For this review, take the finished solid that the model builds, in its own axes (mm). A direction names the side the tool comes from. Round coordinates to 2 decimals unless told otherwise and drop trailing zeros. Order: outer loops, then holes, each group sorted by start corner. A loop starts at its lowest first (then second) coordinate and runs counter-clockwise, first axis right, second up.
Autodesk Inventor part; units mm, degrees
ref_plane "YZ Plane" through (0, 0, 0) normal (1, 0, 0) x (0, 1, 0)
ref_plane "XZ Plane" through (0, 0, 0) normal (0, 1, 0) x (-1, 0, 0)
ref_plane "XY Plane" through (0, 0, 0) normal (0, 0, 1) x (1, 0, 0)
sketch "Sketch1" plane through (0, 0, 0) normal (0, 0, 1) x (1, 0, 0)
  line L0 (0, 0) -> (-34.798, 0)
  line L1 (-34.798, 0) -> (-34.798, -56.642)
  line L2 (0, -12.7) -> (-28.448, -12.7)
  line L3 (-28.448, -12.7) -> (-28.448, -25.654)
  line L4 (-28.448, -25.654) -> (0, -25.654)
  line L5 (0, -56.642) -> (0, -25.654)
  line L6 (0, -12.7) -> (0, 0)
  arc A0 (-7.874, -56.642) -> (-20.574, -56.642) centre (-14.224, -56.642) ccw
  line L7 (-34.798, -56.642) -> (-20.574, -56.642)
  line L8 (-7.874, -56.642) -> (0, -56.642)
  dimension "d0" = 56.642
  dimension "d1" = 34.798
  dimension "d4" = 12.7
  dimension "d5" = 28.448
  dimension "d6" = 12.954
  dimension "d50" = 6.35
  dimension "d51" = 14.224
  dimension "d71" = 56.642
  dimension "d72" = 56.642
extrude "Extrusion4" add sketch "Sketch1" along normal mid plane 12.7
sketch "Sketch9" plane through (-34.798, -56.642, 6.35) normal (-1, 0, 0) x (0, 0, 1)
  line L0 (-12.7, 30.988) -> (0, 30.988) construction
  line L1 (-12.7, 0) -> (-12.7, 6.35) construction
  line L2 (0, 30.988) -> (-12.7, 6.35) construction
  line L3 (0, 6.35) -> (0, 0) construction
  line L4 (0, 6.35) -> (-12.7, 30.988) construction
  line L5 (-6.35, 24.3149) -> (-1.4605, 21.492)
  line L6 (-1.4605, 21.492) -> (-1.4605, 15.846)
  line L7 (-1.4605, 15.846) -> (-6.35, 13.0231)
  line L8 (-6.35, 13.0231) -> (-11.2395, 15.846)
  line L9 (-11.2395, 15.846) -> (-11.2395, 21.492)
  line L10 (-11.2395, 21.492) -> (-6.35, 24.3149)
  line L11 (-12.7, 0) -> (-12.7, 56.642)
  point P0 (-6.35, 56.642)
  point P1 (-6.35, 18.669)
  dimension "d61" = 9.779
extrude "Extrusion5" cut sketch "Sketch9" against normal through all
sketch "Sketch10" plane through (0, 0, -6.35) normal (0, 0, -1) x (-1, 0, 0)
  line L0 (34.798, -40.796) -> (0, -40.796)
  line L1 (34.798, -35.15) -> (0, -35.15)
  line L2 (0, -35.15) -> (34.798, -40.796) construction
  line L3 (34.798, -35.15) -> (0, -35.15) construction
  line L4 (0, -40.796) -> (34.798, -35.15) construction
  point P0 (0, 0)
  point P1 (17.399, -37.973)
hole "Hole6" at (-17.399, -37.973, -6.35) direction (0, 0, 1) diameter 5.1054 end through all
sketch "Sketch11" plane through (-28.448, -25.654, 6.35) normal (1, 0, 0) x (0, 0, -1)
  line L0 (0, -30.988) -> (0, 0) construction
  line L1 (12.7, 12.954) -> (12.7, 0) construction
  line L2 (0, 0) -> (12.7, 12.954) construction
  line L3 (12.7, 12.954) -> (0, 12.954) construction
  line L4 (12.7, 12.954) -> (0, 12.954) construction
  line L5 (0, 12.954) -> (12.7, 0) construction
  point P0 (6.35, 25.654)
  point P1 (6.35, 6.477)
hole "Hole7" at (-28.448, -19.177, 0) direction (-1, 0, 0) diameter 5.1054 end through all
sketch "Sketch12" plane through (-34.798, 0, 6.35) normal (0, 1, 0) x (1, 0, 0)
  line L0 (0, 12.7) -> (0, 0) construction
  point P0 (34.798, 6.35)
  point P1 (25.4, 6.35)
  dimension "d80" = 25.4
hole "Hole8" at (-9.398, 0, 0) direction (0, -1, 0) diameter 5.1054 end up to surface
equation "\"d6\" = slotWidth + printerOffset"
equation "\"d50\" = 0.5 * outsideCylnderDiam"
equation "\"d51\" = centerLineOfCylinder"
equation "\"d52\" = partWidth"
equation "\"d61\" = hexTubing"
equation "\"d62\" = partWidth"
equation "\"centerLineOfCylinder\" = 14.224"
equation "\"slotWidth\" = 12.7"
equation "\"outsideCylnderDiam\" = 12.7"
equation "\"partWidth\" = 12.7"
equation "\"printerOffset\" = 0.254"
properties part number "vexOverSupportForArm"
(1) Add section B-B on x = -10.5. Give the boundary of the cut face in (y, z), plus the area to 3 significant figures.
(2) Add section D-D on y = -51.5. Give the boundary of the cut face in (x, z).
(3) Draft analysis for pull direction Z (two halves, no side actions). For faces 4 (the face through (-17, 0, 0)), 5 (the face through (-11.93, -6.44, -0.33)), 6 (the face through (-18, -28, 6.35)), state which applies: pulls with the +Z half, pulls with the -Z half, needs draft (parallel to the pull), parting line crosses it, or undercut.
(4) Add section A-A on x = -3.5. Give the boundary of the cut face in (y, z), plus the area to 3 significant figures.
(5) Clearance check with flat-ended pins moving along their axes: P1, Ø2, axis at x = -19, z = 3, coming from the -Y side; P2, Ø4.5, axis at x = -17.399, y = -37.973, coming from the -Z side; P3, Ø1, axis at y = -14, z = 0, coming from the +X side; P4, Ø6.5, axis at x = -13.5, z = -2, coming from the -Y side. State where each tip first meets the part, or that it passes through.
(6) Tool access review of faces 1 (the face through (-28.448, -19, 3)), 2 (the face through (-17.643, -42.227, -2.411)), 3 (the face through (0, -45, 0)): name each direction out of +Z, -Z, +X, -X, +Y, -Y from which nothing blocks a thin tool from reaching the whole face with its end or side.
(7) Wall thickness on L1, parallel to X at y = -8, z = 0; L2, parallel to Y at x = -26, z = -5; L3, parallel to Y at x = -27.5, z = 1.5: over which ranges is each line inside the solid? List them lowest first.
(8) Add section C-C on z = 2. Give the boundary of the cut face in (x, y), plus the area to 3 significant figures.
Here are the results:
1. outline: (-51.5, -6.35) - (-25.65, -6.35) - (-25.65, 6.35) - (-51.5, 6.35) - close; (-12.7, -6.35) - (0, -6.35) - (0, -2.3) - (-12.7, -2.3) - close; (-12.7, 2.3) - (0, 2.3) - (0, 6.35) - (-12.7, 6.35) - close; hole (-43.62, 0) - (-40.8, -4.89) - (-35.15, -4.89) - (-32.33, 0) - (-35.15, 4.89) - (-40.8, 4.89) - close
1. area: 348 mm2
2. outline: (-34.8, -6.35) - (-17.95, -6.35) - (-17.95, 6.35) - (-34.8, 6.35) - close; (-10.5, -6.35) - (0, -6.35) - (0, 6.35) - (-10.5, 6.35) - close
3. face 4: needs draft
3. face 5: undercut
3. face 6: pulls with the +Z half
4. outline: (-56.64, -6.35) - (-25.65, -6.35) - (-25.65, 6.35) - (-56.64, 6.35) - close; (-12.7, -6.35) - (0, -6.35) - (0, 6.35) - (-12.7, 6.35) - close; hole (-43.62, 0) - (-40.8, -4.89) - (-35.15, -4.89) - (-32.33, 0) - (-35.15, 4.89) - (-40.8, 4.89) - close
4. area: 472 mm2
5. P1: stops at y = -54
5. P2: passes through
5. P3: stops at x = -28.45
5. P4: stops at y = -51.69
6. face 1: +Z, -Z, +X
6. face 2: +X, -X
6. face 3: +Z, -Z, +X, +Y, -Y
7. L1: x = -34.8 to -11.95, -6.85 to 0
7. L2: y = -56.64 to -25.65, -12.7 to 0
7. L3: y = -56.64 to -42.75, -33.19 to -25.65, -12.7 to 0
8. outline: (-34.8, -56.64) - (-20.57, -56.64) arc R6.35 cw to (-7.87, -56.64) - (0, -56.64) - (0, -42.46) - (-34.8, -42.46) - close; (-34.8, -33.48) - (0, -33.48) - (0, -25.65) - (-28.45, -25.65) - (-28.45, -20.76) - (-34.8, -20.76) - close; (-34.8, -17.59) - (-28.45, -17.59) - (-28.45, -12.7) - (-10.98, -12.7) - (-10.98, 0) - (-34.8, 0) - close; (-7.81, -12.7) - (0, -12.7) - (0, 0) - (-7.81, 0) - close
8. area: 1,170 mm2
